Verification items for this drawing (mm, ordinates from the low corner). Give positions to 0.01 mm unless a question says otherwise; leave off trailing zeros. Loops run counter-clockwise (first coordinate to the right, second up) from the corner with the lowest first, then second, coordinate; pieces in that order, holes last. Notation, with made-up numbers: (60, 43) -> (82, 43) arc R16 cw to (82, 64) -> close; hole circle Ø11 at (48, 66.5). An arc over 180 degrees is marked (long way). Answer as a JSON object with one key per item and string values.
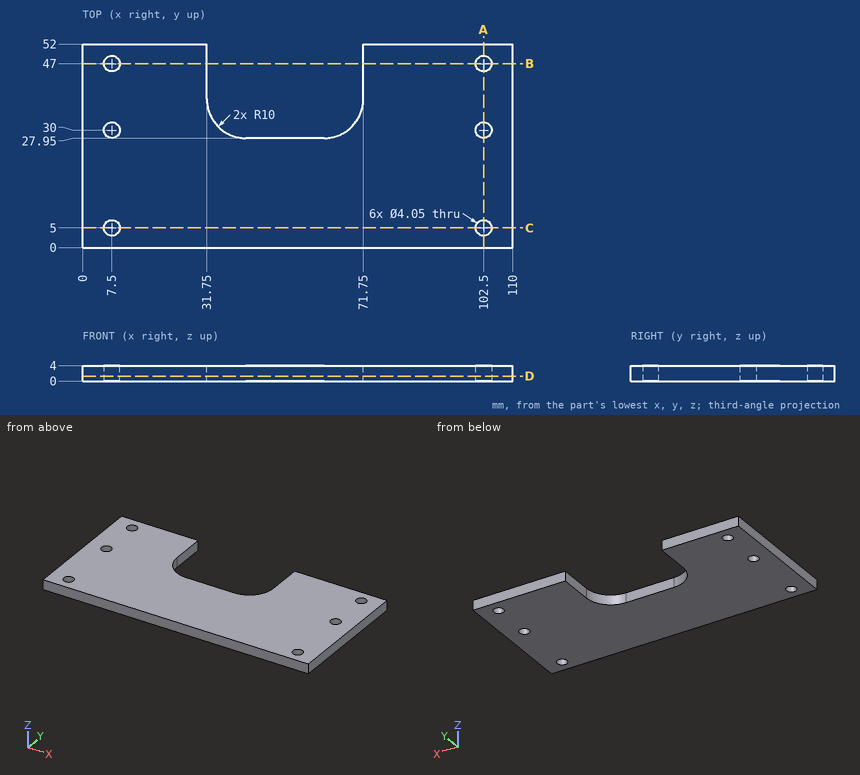
1) Material ranges on line 1 along Y through (x, z) = (102.5, 1.4) (3 decimals); line 2 along X through (y, z) = (35.5, 2.85); line 3 along Y through (x, z) = (62.5, 0.6), recorded low to high. Write a range as from..to.
Geometry check:
{"line 1": "y = 0..2.975, 7.025..27.975, 32.025..44.975, 49.025..52", "line 2": "x = 0..32.05, 71.45..110", "line 3": "y = 0..27.98"}
2) Section check A-A on x = 102.5. Record the cut outline in (y, z) (3 decimals), plus the area to 3 significant figures.
Geometry check:
{"outline": "(0, 0) -> (2.975, 0) -> (2.975, 4) -> (0, 4) -> close; (7.025, 0) -> (27.975, 0) -> (27.975, 4) -> (7.025, 4) -> close; (32.025, 0) -> (44.975, 0) -> (44.975, 4) -> (32.025, 4) -> close; (49.025, 0) -> (52, 0) -> (52, 4) -> (49.025, 4) -> close", "area": "159 mm2"}
3) Section check B-B on y = 47. Record the cut outline in (x, z) (3 decimals).
Geometry check:
{"outline": "(0, 0) -> (5.475, 0) -> (5.475, 4) -> (0, 4) -> close; (9.525, 0) -> (31.75, 0) -> (31.75, 4) -> (9.525, 4) -> close; (71.75, 0) -> (100.475, 0) -> (100.475, 4) -> (71.75, 4) -> close; (104.525, 0) -> (110, 0) -> (110, 4) -> (104.525, 4) -> close"}
4) Section check D-D on z = 1.3. Record the cut outline in (x, y) (3 decimals).
Geometry check:
{"outline": "(0, 0) -> (110, 0) -> (110, 52) -> (71.75, 52) -> (71.75, 37.95) arc R10 cw to (61.75, 27.95) -> (41.75, 27.95) arc R10 cw to (31.75, 37.95) -> (31.75, 52) -> (0, 52) -> close; hole circle Ø4.05 at (7.5, 5); hole circle Ø4.05 at (7.5, 30); hole circle Ø4.05 at (7.5, 47); hole circle Ø4.05 at (102.5, 5); hole circle Ø4.05 at (102.5, 30); hole circle Ø4.05 at (102.5, 47)"}
5) Section check C-C on y = 5. Record the cut outline in (x, z) (3 decimals), plus the area to 3 significant figures.
Geometry check:
{"outline": "(0, 0) -> (5.475, 0) -> (5.475, 4) -> (0, 4) -> close; (9.525, 0) -> (100.475, 0) -> (100.475, 4) -> (9.525, 4) -> close; (104.525, 0) -> (110, 0) -> (110, 4) -> (104.525, 4) -> close", "area": "408 mm2"}
